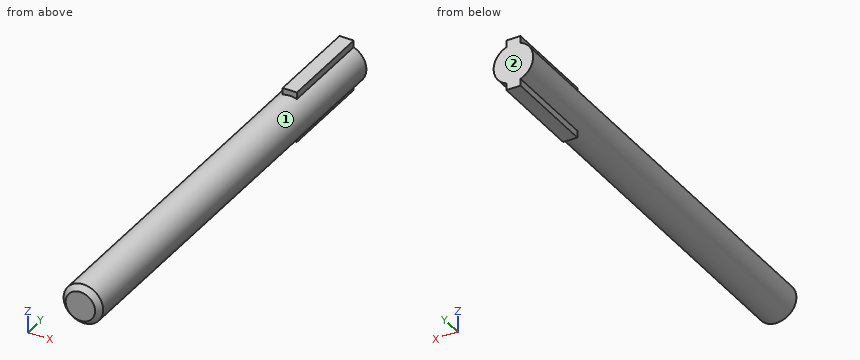
```python
from build123d import *

# Parameters (mm, degrees)
ESQUISSE1_R             = 3.9
BOSS_EXTRU_1_DEPTH      = 8
BOSS_EXTRU_1_DEPTH_BACK = 81
BOSS_EXTRU_2_DEPTH      = 19
CHANFREIN1_SIZE         = 1


with BuildPart() as part:
    # Esquisse1 → Boss.-Extru.1 (new body, two sides)
    with BuildSketch(Plane(origin=(0, 0, 0), x_dir=(1, 0, 0), z_dir=(0, 1, 0))) as boss_extru_1_sk:
        Circle(ESQUISSE1_R)
    extrude(amount=BOSS_EXTRU_1_DEPTH)
    extrude(boss_extru_1_sk.sketch, amount=-BOSS_EXTRU_1_DEPTH_BACK)

    # Esquisse2 → Boss.-Extru.2 (add)
    with BuildSketch(Plane(origin=(0, 8, 0), x_dir=(1, 0, 0), z_dir=(0, 1, 0))):
        with BuildLine():
            Line((-1.4, 5), (-1.4, 3.640054945))
            ThreePointArc((-1.4, 3.640054945), (0, 3.9), (1.4, 3.640054945))
            Line((1.4, 3.640054945), (1.4, 5))
            Line((1.4, 5), (-1.4, 5))
        make_face()
        with BuildLine():
            ThreePointArc((1.4, -3.640054945), (0, -3.9), (-1.4, -3.640054945))
            Line((-1.4, -3.640054945), (-1.4, -5))
            Line((-1.4, -5), (1.4, -5))
            Line((1.4, -5), (1.4, -3.640054945))
        make_face()
        with BuildLine():
            Line((-1.4, 3.640054945), (-1.4, 0))
            Line((-1.4, 0), (1.4, 0))
            Line((1.4, 0), (1.4, 3.640054945))
            ThreePointArc((1.4, 3.640054945), (0, 3.9), (-1.4, 3.640054945))
        make_face()
        with BuildLine():
            Line((1.4, 0), (-1.4, 0))
            Line((-1.4, 0), (-1.4, -3.640054945))
            ThreePointArc((-1.4, -3.640054945), (0, -3.9), (1.4, -3.640054945))
            Line((1.4, -3.640054945), (1.4, 0))
        make_face()
    extrude(amount=-BOSS_EXTRU_2_DEPTH)

    # Chanfrein1
    chanfrein1_edges = [part.edges().sort_by_distance(p)[0] for p in [
        (-3.9, -81, 0),
    ]]
    chamfer(chanfrein1_edges, length=CHANFREIN1_SIZE)


solid = part.part
```
Source: CAD feature listing. Evaluate the final solid. Frame: model axes, mm. Face numbers are marked on the shaded views. A direction names the side the tool comes from. Give positions to 0.01 mm unless a question says otherwise; leave off trailing zeros. Order: outer loops, then holes, each group sorted by start corner. A loop starts at its lowest first (then second) coordinate and runs counter-clockwise, first axis right, second up. Notation, with made-up numbers: (18.25, -36) -> (31.25, -36) arc R29 ccw to (31.25, 0) -> close; hole circle Ø8 at (-20, -8.75). An arc over 180 degrees is marked (long way). Use a Markdown table: item, result.
Q1. Section A-A (x = 0). Return the cut outline in (y, z).
A:
| item | result |
|---|---|
| outline | (-81, -2.9) -> (-80, -3.9) -> (-11, -3.9) -> (-11, -5) -> (8, -5) -> (8, 5) -> (-11, 5) -> (-11, 3.9) -> (-80, 3.9) -> (-81, 2.9) -> close |
Q2. Access query for the marked faces 1 and 2. Directions: +Z, -Z, +X, -X, +Y, -Y. A direction counts if a zero-diameter tool reaches every point of the face in a straight line with its end or side. Return the directions, or none.
A:
| item | result |
|---|---|
| face 1 | -Y |
| face 2 | +Z, -Z, +X, -X, +Y |
Q3. First-contact query: P1, Ø4, axis at x = -1.5, y = -58, coming from the +Z side; P2, Ø1.1, axis at x = 0.5, z = 4, coming from the -Y side; P3, Ø1.1, axis at y = -3.5, z = 4.5, coming from the -X side. Flat tips, straight axial feed; report the tip coordinate or a pass-through.
A:
| item | result |
|---|---|
| P1 | z = 3.9 |
| P2 | y = -80.42 |
| P3 | x = -1.4 |
Q4. Material intervals for line 1 (X direction, y = -8.5, z = 4); line 2 (X direction, y = -5, z = -0.25); line 3 (Y direction, x = -0.25, z = 4.25), sorted ascending. Write a range as [from, to].
A:
| item | result |
|---|---|
| line 1 | [-1.4, 1.4] |
| line 2 | [-3.89, 3.89] |
| line 3 | [-11, 8] |
Q5. Section B-B (y = -66.5). Return the cut outline in (x, z).
A:
| item | result |
|---|---|
| outline | circle Ø7.8 at (0, 0) |
